from build123d import *

# Parameters (mm, degrees)
SKETCH1_W           = 101.6
SKETCH1_H           = 101.6
BOSS_EXTRUDE1_DEPTH = 6.35
SKETCH3_R           = 1.27
CUT_EXTRUDE2_DEPTH  = 7.35
SKETCH4_R           = 1.27
CUT_EXTRUDE3_DEPTH  = 7.35
SKETCH7_R           = 1.89865
CUT_EXTRUDE5_DEPTH  = 7.35
SKETCH8_R           = 1.89865
CUT_EXTRUDE6_DEPTH  = 7.35
SKETCH10_R          = 1.1
CUT_EXTRUDE7_DEPTH  = 7.35


with BuildPart() as part:
    # Sketch1 → Boss-Extrude1 (new body)
    with BuildSketch(Plane(origin=(0, 0, 0), x_dir=(1, 0, 0), z_dir=(0, 1, 0))):
        Rectangle(SKETCH1_W, SKETCH1_H)
    extrude(amount=BOSS_EXTRUDE1_DEPTH)

    # Sketch3 → Cut-Extrude2 (cut, through all)
    with BuildSketch(Plane.XZ):
        with Locations((-8.691546024, 15.75616758)):
            Circle(SKETCH3_R)
        with Locations((-34.262562923, 10.563822948)):
            Circle(SKETCH3_R)
        with Locations((-17.714931052, -9.610745883)):
            Circle(SKETCH3_R)
    extrude(amount=-CUT_EXTRUDE2_DEPTH, mode=Mode.SUBTRACT)

    # Sketch4 → Cut-Extrude3 (cut, through all)
    with BuildSketch(Plane.XZ):
        with Locations((27.2, 41.198822948)):
            Circle(SKETCH4_R)
        with Locations((27.2, -13.721177052)):
            Circle(SKETCH4_R)
    extrude(amount=-CUT_EXTRUDE3_DEPTH, mode=Mode.SUBTRACT)

    # Sketch7 → Cut-Extrude5 (cut, through all)
    with BuildSketch(Plane.XZ):
        with Locations((-32.600738686, -33.3375)):
            Circle(SKETCH7_R)
        with Locations((-32.600738686, 33.3375)):
            Circle(SKETCH7_R)
    extrude(amount=-CUT_EXTRUDE5_DEPTH, mode=Mode.SUBTRACT)

    # Sketch8 → Cut-Extrude6 (cut, through all)
    with BuildSketch(Plane(origin=(0, 6.35, 0), x_dir=(1, 0, 0), z_dir=(0, 1, 0))):
        with Locations((12.280738686, 23.1775)):
            Circle(SKETCH8_R)
    extrude(amount=-CUT_EXTRUDE6_DEPTH, mode=Mode.SUBTRACT)

    # Sketch10 → Cut-Extrude7 (cut, through all)
    with BuildSketch(Plane(origin=(0, 6.35, 0), x_dir=(1, 0, 0), z_dir=(0, 1, 0))):
        with Locations((34.238748138, 43.081855351)):
            Circle(SKETCH10_R)
        with Locations((32.148178872, 23.191417444)):
            Circle(SKETCH10_R)
    extrude(amount=-CUT_EXTRUDE7_DEPTH, mode=Mode.SUBTRACT)


solid = part.part
Verification items for the finished model (mm, model axes). Give positions to 0.01 mm unless a question says otherwise; leave off trailing zeros. Write each loop counter-clockwise with the first axis right and the second up, starting at its lowest first coordinate (ties: lowest second). Pieces come first, ordered by that corner, then holes. Notation, with made-up numbers: M 7,-8 L 52,-8 A17 ccw 52,10 Z; hole C 37.5,-8 d6. An arc over 180 degrees is marked long. Put each result on its own line as item: value. Start each with the question number.
1. Go/stop test with a flat-tipped pin: pin 1 Ø12 at (x, z) = (-21.5, -29.5) entering from -Y. Record where the tip stops, or that it passes through.
2. Scan lines: line 1 along X through (y, z) = (4, -42.5); line 2 along Z through (x, y) = (12, 1.75); line 3 along Z through (x, y) = (-31, 2). Record each from-to range of solid material in increasing order. Write a range as [from, to].
3. Draft check along X on faces 1 (the face through (50.8, 3, 1)), 2 (the face through (-17.99, 3.13, -10.85)), 3 (the face through (-50.8, 3, 1)), 4 (the face through (-1, 6.35, -1)). Enter one of: +X half, -X half, draft (parallel to the pull), parting line (faces both ways), or undercut.
4. Section check A-A (x = 27.2). Record the cut outline in (y, z), and give its area (3 significant figures).
Answer list:
1. pin 1: y = 0
2. line 1: [-50.8, 33.31], [35.17, 50.8]
2. line 2: [-50.8, -25.06], [-21.3, 50.8]
2. line 3: [-50.8, -34.36], [-32.32, 32.32], [34.36, 50.8]
3. face 1: +X half
3. face 2: undercut
3. face 3: -X half
3. face 4: draft
4. outline: M 0,-50.8 L 6.35,-50.8 L 6.35,-14.99 L 0,-14.99 Z; M 0,-12.45 L 6.35,-12.45 L 6.35,39.93 L 0,39.93 Z; M 0,42.47 L 6.35,42.47 L 6.35,50.8 L 0,50.8 Z
4. area: 613 mm2
